from build123d import *

# Parameters (mm, degrees)
SKETCH1_R           = 0.5
SKETCH1_W           = 2
SKETCH1_H           = 2
SKETCH1_H_2         = 6
BOSS_EXTRUDE1_DEPTH = 2
SKETCH2_R           = 1.25
CUT_EXTRUDE1_DEPTH  = 2


with BuildPart() as part:
    # Sketch1 → Boss-Extrude1 (new body)
    # profile 1 of 6: a face of its own
    with BuildSketch(Plane(origin=(0, 4.248778205, 0), x_dir=(1, 0, 0), z_dir=(0, 1, 0))):
        Polygon((12.967182815, 5.558634222), (31.967182815, 5.558634222), (31.967182815, 11.558634222), (27.967182815, 11.558634222), (27.967182815, 7.558634222), (14.967182815, 7.558634222), (14.967182815, 11.558634222), (10.967182815, 11.558634222), (10.967182815, 5.558634222), align=None)
        with Locations(Location((12.967182815, 9.558634222, 0), (0, 0, 270))):
            Circle(SKETCH1_R, mode=Mode.SUBTRACT)
        with Locations(Location((29.967182815, 9.558634222, 0), (0, 0, 270))):
            Circle(SKETCH1_R, mode=Mode.SUBTRACT)
    # profile 2 of 6: a face of its own
    with BuildSketch(Plane(origin=(0, 4.248778205, 0), x_dir=(1, 0, 0), z_dir=(0, 1, 0))):
        Polygon((31.967182815, -0.441365778), (31.967182815, 5.558634222), (12.967182815, 5.558634222), (12.967182815, 3.558634222), (10.967182815, 3.558634222), (10.967182815, -4.441365778), (12.967182815, -4.441365778), (12.967182815, -6.441365778), (29.967182815, -6.441365778), (29.967182815, -0.441365778), align=None)
    # profile 3 of 6: a face of its own
    with BuildSketch(Plane(origin=(0, 4.248778205, 0), x_dir=(1, 0, 0), z_dir=(0, 1, 0))):
        Polygon((31.967182815, -12.441365778), (31.967182815, -6.441365778), (29.967182815, -6.441365778), (12.967182815, -6.441365778), (10.967182815, -6.441365778), (10.967182815, -12.441365778), (14.967182815, -12.441365778), (14.967182815, -8.441365778), (27.967182815, -8.441365778), (27.967182815, -12.441365778), align=None)
        with Locations(Location((12.967182815, -10.441365778, 0), (0, 0, 270))):
            Circle(SKETCH1_R, mode=Mode.SUBTRACT)
        with Locations(Location((29.967182815, -10.441365778, 0), (0, 0, 270))):
            Circle(SKETCH1_R, mode=Mode.SUBTRACT)
    # profile 4 of 6: a face of its own
    with BuildSketch(Plane(origin=(0, 4.248778205, 0), x_dir=(1, 0, 0), z_dir=(0, 1, 0))):
        with Locations((11.967182815, -5.441365778)):
            Rectangle(SKETCH1_W, SKETCH1_H)
    # profile 5 of 6: a face of its own
    with BuildSketch(Plane(origin=(0, 4.248778205, 0), x_dir=(1, 0, 0), z_dir=(0, 1, 0))):
        with Locations((11.967182815, 4.558634222)):
            Rectangle(SKETCH1_W, SKETCH1_H)
    # profile 6 of 6: a face of its own
    with BuildSketch(Plane(origin=(0, 4.248778205, 0), x_dir=(1, 0, 0), z_dir=(0, 1, 0))):
        with Locations((30.967182815, -3.441365778)):
            Rectangle(SKETCH1_W, SKETCH1_H_2)
    extrude(amount=BOSS_EXTRUDE1_DEPTH)

    # Sketch2 → Cut-Extrude1 (cut)
    with BuildSketch(Plane(origin=(0, 6.248778205, 0), x_dir=(1, 0, 0), z_dir=(0, 1, 0))):
        with Locations(Location((28.672843406, -5.034622275, 0), (0, 0, 270))):
            Circle(SKETCH2_R)
    extrude(amount=-CUT_EXTRUDE1_DEPTH, mode=Mode.SUBTRACT)


solid = part.part
The model under review builds one solid part; all positions refer to its coordinate system, in mm. A direction names the side the tool comes from. Round coordinates to 2 decimals unless told otherwise and drop trailing zeros. Loops run counter-clockwise (first coordinate to the right, second up) from the corner with the lowest first, then second, coordinate; pieces in that order, holes last. Notation, with made-up numbers: (29.5, 0.25) -> (44.5, 0.25) arc R25 ccw to (44.5, 12.25) -> close; hole circle Ø11 at (37, -7.5). An arc over 180 degrees is marked (long way). Answer as CSV lines item,"result".
1) Draft analysis for pull direction X (two halves, no side actions). For faces 1 (the face through (31.967, 5, 1)), 2 (the face through (29.91, 5.26, 4.87)), 3 (the face through (13, 5, 12.441)), 4 (the face through (12.524, 5.235, -9.328)), state which applies: pulls with the +X half, pulls with the -X half, needs draft (parallel to the pull), parting line crosses it, or undercut.
Geometry results:
face 1,"pulls with the +X half"
face 2,"undercut"
face 3,"needs draft"
face 4,"undercut"
2) Add section B-B on y = 5.2. Write out the cut boundary in (x, z), plus the area to 3 significant figures.
Geometry results:
outline,"(10.97, -11.56) -> (14.97, -11.56) -> (14.97, -7.56) -> (27.97, -7.56) -> (27.97, -11.56) -> (31.97, -11.56) -> (31.97, 12.44) -> (27.97, 12.44) -> (27.97, 8.44) -> (14.97, 8.44) -> (14.97, 12.44) -> (10.97, 12.44) -> close; hole circle Ø1 at (12.97, -9.56); hole circle Ø1 at (12.97, 10.44); hole circle Ø2.5 at (28.67, 5.03); hole circle Ø1 at (29.97, -9.56); hole circle Ø1 at (29.97, 10.44)"
area,"392 mm²"
3) Add section D-D on x = 17.25. Write out the cut boundary in (y, z).
Geometry results:
outline,"(4.25, -7.56) -> (6.25, -7.56) -> (6.25, 8.44) -> (4.25, 8.44) -> close"
4) To check wall thickness, follow line 1 along X through (y, z) = (5.25, 5); line 2 along Z through (x, y) = (29.75, 5.2); line 3 along X through (y, z) = (5.7, -7.75). State the ranges of each line that lie inside material, in increasing order. Write a range as from..to.
Geometry results:
line 1,"x = 10.97..27.42, 29.92..31.97"
line 2,"z = -11.56..-10.01, -9.11..4.4, 5.67..9.99, 10.89..12.44"
line 3,"x = 10.97..14.97, 27.97..31.97"
5) Add section C-C on z = 4.5. Write out the cut boundary in (x, y), plus the area to 3 significant figures.
Geometry results:
outline,"(10.97, 4.25) -> (27.54, 4.25) -> (27.54, 6.25) -> (10.97, 6.25) -> close; (29.8, 4.25) -> (31.97, 4.25) -> (31.97, 6.25) -> (29.8, 6.25) -> close"
area,"37.5 mm²"
6) Tool access review of faces 5 (the face through (21, 5, 8.441)), 6 (the face through (10.967, 5, 0)), 7 (the face through (27.967, 5, -10)): name each direction out of +Z, -Z, +X, -X, +Y, -Y from which nothing blocks a thin tool from reaching the whole face with its end or side.
Geometry results:
face 5,"+Z, +Y, -Y"
face 6,"+Z, -Z, -X, +Y, -Y"
face 7,"-Z, +Y, -Y"
7) For P1, Ø0.6, axis at x = 20, y = 5, coming from the +Z side; P2, Ø4, axis at x = 28.67, z = 5.03, coming from the -Y side; P3, Ø0.6, axis at x = 22.5, y = 5.5, coming from the -Z side, all flat-tipped, find the tip position at first contact; note any pin that passes through.
Geometry results:
P1,"stops at z = 8.44"
P2,"stops at y = 4.25"
P3,"stops at z = -7.56"
8) Add section A-A on z = -8.25. Write out the cut boundary in (x, y).
Geometry results:
outline,"(10.97, 4.25) -> (14.97, 4.25) -> (14.97, 6.25) -> (10.97, 6.25) -> close; (27.97, 4.25) -> (31.97, 4.25) -> (31.97, 6.25) -> (27.97, 6.25) -> close"
